Work out the finished part from the listing and answer in its coordinate system (mm). Face numbers are marked on the shaded views. A direction names the side the tool comes from. Give positions to 0.01 mm unless a question says otherwise; leave off trailing zeros. Loops run counter-clockwise (first coordinate to the right, second up) from the corner with the lowest first, then second, coordinate; pieces in that order, holes last. Notation, with made-up numbers: M 34.5,-37 L 80.5,-37 A7 cw 80.5,-28 Z; hole C -3.5,48 d2. An arc over 180 degrees is marked long. Write item = value, one per line. Start each with the question number.
1. Section B-B on y = 12 is taken. Determine the outline of the cut face in (x, z).
2. Consider L1, parallel to Z at x = 0, y = 5.5; L2, parallel to Y at x = 8.5, z = 9; L3, parallel to X at y = 18, z = 7. Determine where each line is inside the solid, lowest interval first. Write a range as [from, to].
3. Section A-A on x = 0 is taken. Determine the outline of the cut face in (y, z).
4. Section C-C on z = 0 is taken. Determine the outline of the cut face in (x, y).
5. For the marked faces 1 and 2, determine the directions among +Z, -Z, +X, -X, +Y, -Y from which every point of the face is accessible in a straight line to the end or side of a thin tool.
```python
from build123d import *

# Parameters (mm, degrees)
F0_W     = 203.2
F0_H     = 127
F1_DEPTH = 25.4
F2_W     = 203.2
F2_H     = 127
F2_R     = 12.7
F3_DEPTH = 25.4


with BuildPart() as f1:
    # F0 (on Front) → F1 (new body)
    with BuildSketch(Plane.XZ):
        Rectangle(F0_W, F0_H)
    extrude(amount=F1_DEPTH)

    # F2 (on face) → F3 (join)
    with BuildSketch(Plane(origin=(0, 0, 0), x_dir=(-1, 0, 0), z_dir=(0, 1, 0))):
        Rectangle(F2_W, F2_H)
        Circle(F2_R, mode=Mode.SUBTRACT)
    extrude(amount=F3_DEPTH)


solid = f1.part
```
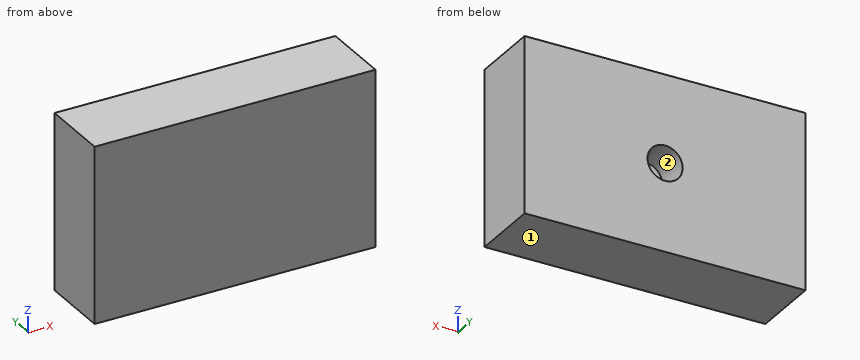
Verdict:
q1.outline = M -101.6,-63.5 L 101.6,-63.5 L 101.6,63.5 L -101.6,63.5 Z; hole C 0,0 d25.4
q2.L1 = [-63.5, -12.7], [12.7, 63.5]
q2.L2 = [-25.4, 0]
q2.L3 = [-101.6, -10.6], [10.6, 101.6]
q3.outline = M -25.4,-63.5 L 25.4,-63.5 L 25.4,-12.7 L 0,-12.7 L 0,12.7 L 25.4,12.7 L 25.4,63.5 L -25.4,63.5 Z
q4.outline = M -101.6,-25.4 L 101.6,-25.4 L 101.6,25.4 L 12.7,25.4 L 12.7,0 L -12.7,0 L -12.7,25.4 L -101.6,25.4 Z
q5.face_1 = -Z, +X, -X, +Y, -Y
q5.face_2 = +Y
